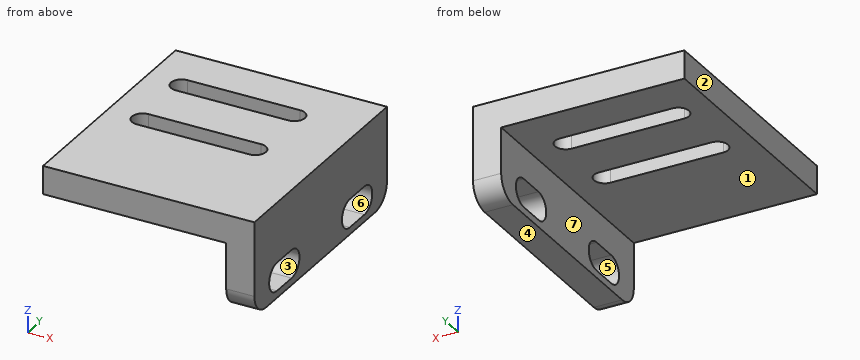
from build123d import *

# Parameters (mm, degrees)
F1_DEPTH = 4
F2_W     = 4
F2_H     = 34
F2_W_2   = 26
F3_DEPTH = 4


# Not quite as in the source:
# - a feature names something its author has since deleted; it is built from what else it names


with BuildPart() as f1:
    # F0 (on Right) → F1 (new body)
    with BuildSketch(Plane.YZ):
        with BuildLine():
            ThreePointArc((-3, 29.5474529266), (-2.1213203436, 31.6687732702), (0, 32.5474529266))
            Line((0, 32.5474529266), (28, 32.5474529266))
            ThreePointArc((28, 32.5474529266), (30.1213203436, 31.6687732702), (31, 29.5474529266))
            Line((31, 29.5474529266), (31, 36.0474529266))
            Line((31, 36.0474529266), (-3, 36.0474529266))
            Line((-3, 36.0474529266), (-3, 29.5474529266))
        make_face()
        with BuildLine():
            Line((28, 32.5474529266), (0, 32.5474529266))
            ThreePointArc((0, 32.5474529266), (-2.1213203436, 31.6687732702), (-3, 29.5474529266))
            ThreePointArc((-3, 29.5474529266), (-2.1213203436, 27.4261325831), (0, 26.5474529266))
            Line((0, 26.5474529266), (28, 26.5474529266))
            ThreePointArc((28, 26.5474529266), (30.1213203436, 27.4261325831), (31, 29.5474529266))
            ThreePointArc((31, 29.5474529266), (30.1213203436, 31.6687732702), (28, 32.5474529266))
        make_face()
        with BuildLine():
            ThreePointArc((2.7801140677, 27.5474529266), (0.7801140677, 29.5474529266), (2.7801140677, 31.5474529266))
            Line((2.7801140677, 31.5474529266), (6.5496175084, 31.5474529266))
            ThreePointArc((6.5496175084, 31.5474529266), (8.5496175084, 29.5474529266), (6.5496175084, 27.5474529266))
            Line((6.5496175084, 27.5474529266), (2.7801140677, 27.5474529266))
        make_face(mode=Mode.SUBTRACT)
        with BuildLine():
            Line((21.4503824916, 31.5474529266), (25.2198859323, 31.5474529266))
            ThreePointArc((25.2198859323, 31.5474529266), (27.2198859323, 29.5474529266), (25.2198859323, 27.5474529266))
            Line((25.2198859323, 27.5474529266), (21.4503824916, 27.5474529266))
            ThreePointArc((21.4503824916, 27.5474529266), (19.4503824916, 29.5474529266), (21.4503824916, 31.5474529266))
        make_face(mode=Mode.SUBTRACT)
    extrude(amount=-F1_DEPTH)

    # F2 (on face) → F3 (join)
    with BuildSketch(Plane.XY.offset(36.0474529266)):
        with Locations((-2, 14)):
            Rectangle(F2_W, F2_H)
        with Locations((-17, 14)):
            Rectangle(F2_W_2, F2_H)
        with BuildLine():
            ThreePointArc((-9, 15), (-7.5, 13.5), (-9, 12))
            Line((-9, 12), (-25, 12))
            ThreePointArc((-25, 12), (-26.5, 13.5), (-25, 15))
            Line((-25, 15), (-9, 15))
        make_face(mode=Mode.SUBTRACT)
        with BuildLine():
            ThreePointArc((-9, 25), (-7.5, 23.5), (-9, 22))
            Line((-9, 22), (-25, 22))
            ThreePointArc((-25, 22), (-26.5, 23.5), (-25, 25))
            Line((-25, 25), (-9, 25))
        make_face(mode=Mode.SUBTRACT)
    extrude(amount=F3_DEPTH)


solid = f1.part
CAD build for the part. Positions are in the model's coordinates, mm. Face numbers are marked on the shaded views. A direction names the side the tool comes from. Round coordinates to 2 decimals unless told otherwise and drop trailing zeros. Write each loop counter-clockwise with the first axis right and the second up, starting at its lowest first coordinate (ties: lowest second). Pieces come first, ordered by that corner, then holes. Notation, with made-up numbers: M 46,68 L 52,68 A22 ccw 52,86 Z; hole C 17.5,34 d10. An arc over 180 degrees is marked long. Use a Markdown table: item, result. Add a question column.
1. Slice it at B-B on y = 23.5. Give the cut face in (x, z), then the cut area to 3 significant figures.
2. Slice it at A-A on z = 37.75. Give the cut face in (x, y).
3. 3-axis set-ups, long thin cutter, end or side, ignore diameter. For the marked faces 1, 2 and 3: which of +Z, -Z, +X, -X, +Y, -Y reach the whole face in a straight line?
4. Slice it at C-C on x = -16. Give the cut face in (y, z).
5. Flat gauge pins, fed straight in: P1, Ø8, axis at x = -23, y = 2.5, coming from the -Z side; P2, Ø5, axis at y = 11.5, z = 30, coming from the -X side. Where does each tip first touch, or does it go through?
6. Pull direction Z, two halves, no side cores. Call the marked faces 4, 5, 6 and 7: released by +Z, released by -Z, zero draft, split by the parting line, or undercut.
7. Slice it at D-D on y = 12.5. Give the cut face in (x, z), then the cut area to 3 significant figures.
8. Drill centre lines: probe 1 along Y at (x, z) = (-25, 38); probe 2 along Y at (x, z) = (-2, 28.75); probe 3 along X at (y, z) = (20, 33.75). Where is each one in solid material? Low to high.
Reply:
| question | item | result |
|---|---|---|
| 1 | outline | M -30,36.05 L -26.5,36.05 L -26.5,40.05 L -30,40.05 Z; M -7.5,36.05 L -4,36.05 L -4,31.55 L 0,31.55 L 0,40.05 L -7.5,40.05 Z; M -4,26.55 L 0,26.55 L 0,27.55 L -4,27.55 Z |
| 1 | area | 66.0 mm^2 |
| 2 | outline | M -30,-3 L 0,-3 L 0,31 L -30,31 Z; hole M -25,12 L -9,12 A1.5 ccw -9,15 L -25,15 A1.5 ccw Z; hole M -25,22 L -9,22 A1.5 ccw -9,25 L -25,25 A1.5 ccw Z |
| 3 | face 1 | -Z, -X, +Y, -Y |
| 3 | face 2 | +Z, -Z, -X, +Y, -Y |
| 3 | face 3 | +X, -X |
| 4 | outline | M -3,36.05 L 12,36.05 L 12,40.05 L -3,40.05 Z; M 15,36.05 L 22,36.05 L 22,40.05 L 15,40.05 Z; M 25,36.05 L 31,36.05 L 31,40.05 L 25,40.05 Z |
| 5 | P1 | stops at z = 36.05 |
| 5 | P2 | stops at x = -4 |
| 6 | face 4 | released by -Z |
| 6 | face 5 | undercut |
| 6 | face 6 | undercut |
| 6 | face 7 | zero draft |
| 7 | outline | M -30,36.05 L -26.12,36.05 L -26.12,40.05 L -30,40.05 Z; M -7.88,36.05 L -4,36.05 L -4,26.55 L 0,26.55 L 0,40.05 L -7.88,40.05 Z |
| 7 | area | 85.1 mm^2 |
| 8 | probe 1 | y = -3 to 12, 15 to 22, 25 to 31 |
| 8 | probe 2 | y = -2.89 to 0.95, 8.38 to 19.62, 27.05 to 30.89 |
| 8 | probe 3 | x = -4 to 0 |
